Can you work these out from the model? Positions are in its coordinate system, mm. A direction names the side the tool comes from. Coordinates: 2 decimals unless noted, no trailing zeros. Loops run counter-clockwise (first coordinate to the right, second up) from the corner with the lowest first, then second, coordinate; pieces in that order, holes last.
```python
from build123d import *

# Parameters (mm, degrees)
F1_DEPTH = 6.35
F2_W     = 25.4
F2_H     = 6.35
F3_DEPTH = 9.525
F4_R     = 5.08


with BuildPart() as f1:
    # F0 (on Front) → F1 (new body)
    with BuildSketch(Plane.XZ):
        with BuildLine():
            Line((-9.525, -9.525), (9.525, -9.525))
            Line((9.525, -9.525), (15.875, -9.525))
            Line((15.875, -9.525), (41.275, -9.525))
            Line((41.275, -9.525), (41.275, 9.525))
            Line((41.275, 9.525), (15.875, 9.525))
            Line((15.875, 9.525), (9.525, 9.525))
            Line((9.525, 9.525), (0, 9.525))
            ThreePointArc((0, 9.525), (-6.735192, 6.735192), (-9.525, 0))
            Line((-9.525, 0), (-9.525, -9.525))
        make_face()
    extrude(amount=F1_DEPTH)

    # F2 (on Top) → F3 (join, symmetric)
    with BuildSketch(Plane.XY):
        with Locations((28.575, 3.175)):
            Rectangle(F2_W, F2_H)
        Polygon((-123.825, 6.35), (15.875, 6.35), (41.275, 6.35), (41.275, 12.7), (-123.825, 12.7), align=None)
    extrude(amount=F3_DEPTH, both=True)

    # F4
    f4_edges = [f1.edges().sort_by_distance(p)[0] for p in [
        (-123.825, 12.7, 0),
    ]]
    fillet(f4_edges, radius=F4_R)


solid = f1.part
```
(1) Which directions (+Z, -Z, +X, -X, +Y, -Y) give clear straight access to the entire face, cutting with the end or side of a thin tool? Please do faces 1 (the flat face through (-24, 8, 9.525)), 2 (the flat face through (-9.525, -3, -5)), 3 (the cylindrical face through (-122.38, 11.17, -0.13)), 4 (the cylindrical face through (-6.66, -3.13, 6.81)), 5 (the flat face through (-55, 6.35, 0)).
Check values:
face 1: +Z, +X, -X, +Y, -Y
face 2: +Z, -Z, -X, -Y
face 3: +Z, -Z, -X, +Y
face 4: +Z, -X, -Y
face 5: +Z, -Z, -X
(2) If I drill on probe 1 along Y at (x, z) = (15.5, 1); probe 2 along Y at (x, z) = (-20.5, 2); probe 3 along X at (y, z) = (6.25, 8.5) (3 decimals), over which ranges is the centre line in solid material (lowest first)?
Check values:
probe 1: y = -6.35 to 0, 6.35 to 12.7
probe 2: y = 6.35 to 12.7
probe 3: x = 15.875 to 41.275
(3) I'm going to push flat-ended pins straight in: pin 1 (5.5 mm diameter, centred on x = -44, z = -4.5, fed in from -Y); pin 2 (1.9 mm diameter, centred on y = -2, z = -4, fed in from -X) (3 decimals); pin 3 (3 mm diameter, centred on y = 3.5, z = 4.5, fed in from -X) (3 decimals). Where does each tip first touch, or does it pass through?
Check values:
pin 1: stops at y = 6.35
pin 2: stops at x = -9.525
pin 3: stops at x = 15.875
(4) I want a section at B-B on x = -64. Write out the boundary of the cut face in (y, z) (3 decimals).
Check values:
outline: (6.35, -9.525) - (12.7, -9.525) - (12.7, 9.525) - (6.35, 9.525) - close
(5) I want a section at D-D on z = 6.5. Write out the boundary of the cut face in (x, y) (3 decimals), then the cut area to 3 significant figures.
Check values:
outline: (-123.825, 6.35) - (15.875, 6.35) - (15.875, 0) - (-6.962, 0) - (-6.962, -6.35) - (41.275, -6.35) - (41.275, 12.7) - (-118.745, 12.7) arc R5.08 ccw to (-123.825, 7.62) - close
area: 1,510 mm2
(6) If we mould it in two halves opening along Y, with no side actions, what happens to faces 6 (the flat face through (16, -6.35, 0)), 7 (the flat face through (-38, 12.7, 0)), 8 (the flat face through (15.875, 3, 0)), 9 (the flat face through (3, 0, 0))? For each: released by +Y, released by -Y, zero draft, split by the parting line, or undercut.
Check values:
face 6: released by -Y
face 7: released by +Y
face 8: undercut
face 9: undercut
(7) I want a section at C-C on y = 1.75. Write out the boundary of the cut face in (x, z) (3 decimals).
Check values:
outline: (15.875, -9.525) - (41.275, -9.525) - (41.275, 9.525) - (15.875, 9.525) - close
(8) I want a section at A-A on z = -2.5. Write out the boundary of the cut face in (x, y) (3 decimals), then the cut area to 3 significant figures.
Check values:
outline: (-123.825, 6.35) - (15.875, 6.35) - (15.875, 0) - (-9.525, 0) - (-9.525, -6.35) - (41.275, -6.35) - (41.275, 12.7) - (-118.745, 12.7) arc R5.08 ccw to (-123.825, 7.62) - close
area: 1,530 mm2
